The listing builds one solid part. Answer for the finished solid, in the listing's coordinates (mm). A direction names the side the tool comes from. Round coordinates to 2 decimals unless told otherwise and drop trailing zeros. Loops run counter-clockwise (first coordinate to the right, second up) from the corner with the lowest first, then second, coordinate; pieces in that order, holes last. Notation, with made-up numbers: M 38,-35.75 L 55,-35.75 A30 cw 55,3.25 Z; hole C 3.25,-19.5 d6. An arc over 180 degrees is marked long. Answer as a JSON object with one key per item and string values.
```python
from build123d import *

# Parameters (mm, degrees)
SKETCH_1_R          = 2
SKETCH_1_W          = 41
SKETCH_1_H          = 20
EXTRUDE_1_DEPTH     = 4.4
SKETCH_2_R          = 2.5
CUT_EXTRUDE_1_DEPTH = 4.4


with BuildPart() as part:
    # 草图1 → 凸台-拉伸1 (new body)
    with BuildSketch(Plane.XY):
        Polygon((9, 15), (9, 19.4), (24, 19.4), (24, 15), (36.5, 15), (36.5, -15), (24, -15), (24, -19.4), (9, -19.4), (9, -15), (-9, -15), (-9, -19.4), (-24, -19.4), (-24, -15), (-36.5, -15), (-36.5, 15), (-24, 15), (-24, 19.4), (-9, 19.4), (-9, 15), align=None)
        with Locations((-32, 5)):
            Circle(SKETCH_1_R, mode=Mode.SUBTRACT)
        with Locations((-32, -5)):
            Circle(SKETCH_1_R, mode=Mode.SUBTRACT)
        with Locations((17, -5)):
            Circle(SKETCH_1_R, mode=Mode.SUBTRACT)
        with Locations((17, 5)):
            Circle(SKETCH_1_R, mode=Mode.SUBTRACT)
        with Locations((-7.5, 0)):
            Rectangle(SKETCH_1_W, SKETCH_1_H, mode=Mode.SUBTRACT)
    extrude(amount=EXTRUDE_1_DEPTH)

    # 草图2 → 切除-拉伸1 (cut)
    with BuildSketch(Plane.XY.offset(4.4)):
        with Locations((-28, 0)):
            Circle(SKETCH_2_R)
    extrude(amount=-CUT_EXTRUDE_1_DEPTH, mode=Mode.SUBTRACT)


solid = part.part
```
Item 1: The part is cut by section D-D (y = 16.5). Give the vertices of the cut face in (x, z).
Values follow:
{"outline": "M -24,0 L -9,0 L -9,4.4 L -24,4.4 Z; M 9,0 L 24,0 L 24,4.4 L 9,4.4 Z"}
Item 2: Determine the mould class of faces 4 (the face through (-9, 17, 2)), 5 (the face through (16, 19.4, 2)), 6 (the face through (-28, -6, 2)) for opening direction Y: released by +Y, released by -Y, zero draft, split by the parting line, or undercut.
Values follow:
{"face 4": "zero draft", "face 5": "released by +Y", "face 6": "undercut"}
Item 3: Flat-ended cylindrical pins translate along their axes: P1, Ø1.5, axis at x = 28, z = 3, coming from the -Y side; P2, Ø1.3, axis at y = 18, z = 2, coming from the +X side; P3, Ø1.3, axis at x = -29.5, z = 2, coming from the +Y side. Find the tip coordinate at first contact, or state that the pin passes through.
Values follow:
{"P1": "y = -15", "P2": "x = 24", "P3": "y = 15"}
Item 4: Straight lines are drawn through the part: line 1 (Y direction, x = 17, z = 3); line 2 (Y direction, x = -32, z = 3.4); line 3 (X direction, y = -5.5, z = 0.2). For each, find the intervals that lie inside material, in ascending order.
Values follow:
{"line 1": "-19.4 to -7, -3 to 3, 7 to 19.4", "line 2": "-15 to -7, -3 to 3, 7 to 15", "line 3": "-36.5 to -33.94, -30.06 to -28, 13 to 15.06, 18.94 to 36.5"}
Item 5: The part is cut by section C-C (x = -32). Give the vertices of the cut face in (y, z).
Values follow:
{"outline": "M -15,0 L -7,0 L -7,4.4 L -15,4.4 Z; M -3,0 L 3,0 L 3,4.4 L -3,4.4 Z; M 7,0 L 15,0 L 15,4.4 L 7,4.4 Z"}
Item 6: Which of the six approach directions +Z, -Z, +X, -X, +Y, -Y give full straight-line access (tool end or side, diameter ignored) to faces 1 (the face through (-30, 15, 2)), 2 (the face through (24, 17, 2)), 3 (the face through (-9, -17, 2))?
Values follow:
{"face 1": "+Z, -Z, -X, +Y", "face 2": "+Z, -Z, +X, +Y", "face 3": "+Z, -Z, -Y"}
Item 7: The part is cut by section A-A (y = 5). Give the vertices of the cut face in (x, z).
Values follow:
{"outline": "M -36.5,0 L -34,0 L -34,4.4 L -36.5,4.4 Z; M -30,0 L -28,0 L -28,4.4 L -30,4.4 Z; M 13,0 L 15,0 L 15,4.4 L 13,4.4 Z; M 19,0 L 36.5,0 L 36.5,4.4 L 19,4.4 Z"}
Item 8: The part is cut by section B-B (z = 2.95). Give the number of separate pieces and of enclosed holes in the cut face, then the cut area to 3 significant figures.
Values follow:
{"separate pieces": "1", "enclosed holes": "5", "area": "1,570 mm^2"}
